Could you check a few things on this model? Use its own coordinates, in mm. A direction names the side the tool comes from. Round coordinates to 2 decimals unless told otherwise and drop trailing zeros. Write each loop counter-clockwise with the first axis right and the second up, starting at its lowest first coordinate (ties: lowest second). Pieces come first, ordered by that corner, then holes. Notation, with made-up numbers: (19, 78) -> (62, 78) arc R17 cw to (62, 84) -> close; hole circle Ø1 at (52.5, -30.75). An arc over 180 degrees is marked (long way). Answer in a Markdown table with one row per item. Add a question column.
```python
from build123d import *

# Parameters (mm, degrees)
SKETCH_W        = 40
SKETCH_H        = 35
PAD_DEPTH       = 40
SKETCH001_R     = 12.5
POCKET_DEPTH    = 40.001
SKETCH002_W     = 24.731892
SKETCH002_H     = 24.731892
POCKET001_DEPTH = 35
POCKET002_DEPTH = 35
SKETCH004_W     = 2.5
SKETCH004_H     = 30
POCKET003_DEPTH = 40.001
SKETCH005_W     = 2.5
SKETCH005_H     = 30
POCKET004_DEPTH = 21
SKETCH006_W     = 39.144078
SKETCH006_H     = 33.985684
PAD001_DEPTH    = 3
SKETCH007_W     = 18
SKETCH007_H     = 2
POCKET005_DEPTH = 5
SKETCH008_W     = 2.5
SKETCH008_H     = 15
POCKET006_DEPTH = 1.5
SKETCH009_W     = 21
SKETCH009_H     = 2.5
POCKET007_DEPTH = 1.5


with BuildPart() as part:
    # Sketch → Pad (new body)
    with BuildSketch(Plane.XY):
        with Locations((0, -2.5)):
            Rectangle(SKETCH_W, SKETCH_H)
    extrude(amount=PAD_DEPTH)

    # Sketch001 (on Face5 of Pad) → Pocket (cut, through all)
    with BuildSketch(Plane(origin=(0, 0, 0), x_dir=(1, 0, 0), z_dir=(0, 0, -1))):
        Circle(SKETCH001_R)
    extrude(amount=-POCKET_DEPTH, mode=Mode.SUBTRACT)

    # Sketch002 (on Face5 of Pocket) → Pocket001 (cut)
    with BuildSketch(Plane.XY.offset(40)):
        Rectangle(SKETCH002_W, SKETCH002_H)
    extrude(amount=-POCKET001_DEPTH, mode=Mode.SUBTRACT)

    # Sketch003 → Pocket002 (cut)
    with BuildSketch(Plane.XY.offset(40)):
        Polygon((-18.24138, 13.149356), (-15.24138, 13.149356), (-15.24138, -15.688641), (15.24138, -15.688641), (15.24138, 12.981641), (18.24138, 12.981641), (18.24138, -18.180522), (-18.24138, -18.180522), align=None)
    extrude(amount=-POCKET002_DEPTH, mode=Mode.SUBTRACT)

    # Sketch004 → Pocket003 (cut, through all)
    with BuildSketch(Plane.YZ.offset(20)):
        with Locations((-10.75, 20)):
            Rectangle(SKETCH004_W, SKETCH004_H)
        with Locations((-5.25, 20)):
            Rectangle(SKETCH004_W, SKETCH004_H)
        with Locations((0.25, 20)):
            Rectangle(SKETCH004_W, SKETCH004_H)
        with Locations((5.75, 20)):
            Rectangle(SKETCH004_W, SKETCH004_H)
    extrude(amount=-POCKET003_DEPTH, mode=Mode.SUBTRACT)

    # Sketch005 → Pocket004 (cut)
    with BuildSketch(Plane.XZ.offset(20)):
        with Locations((-5.5, 20)):
            Rectangle(SKETCH005_W, SKETCH005_H)
        with Locations((0, 20)):
            Rectangle(SKETCH005_W, SKETCH005_H)
        with Locations((5.5, 20)):
            Rectangle(SKETCH005_W, SKETCH005_H)
        with Locations((11, 20)):
            Rectangle(SKETCH005_W, SKETCH005_H)
        with Locations((-11, 20)):
            Rectangle(SKETCH005_W, SKETCH005_H)
    extrude(amount=-POCKET004_DEPTH, mode=Mode.SUBTRACT)

    # Sketch006 → Pad001 (join)
    with BuildSketch(Plane.XY.offset(40)):
        with Locations((0.008508, -2.623403)):
            Rectangle(SKETCH006_W, SKETCH006_H)
    extrude(amount=-PAD001_DEPTH)

    # Sketch007 (on Face89 of Pad001) → Pocket005 (cut)
    with BuildSketch(Plane.XY.offset(5)):
        with Locations((0, 5.022821)):
            Rectangle(SKETCH007_W, SKETCH007_H)
        Rectangle(SKETCH007_W, SKETCH007_H)
        with Locations((0, -5.022821)):
            Rectangle(SKETCH007_W, SKETCH007_H)
    extrude(amount=-POCKET005_DEPTH, mode=Mode.SUBTRACT)

    # Sketch008 (on Face117 of Pocket005) → Pocket006 (cut)
    with BuildSketch(Plane.XY.offset(40)):
        with Locations((-8.25, 0)):
            Rectangle(SKETCH008_W, SKETCH008_H)
        with Locations((8.25, 0)):
            Rectangle(SKETCH008_W, SKETCH008_H)
        with Locations((-2.75, 0)):
            Rectangle(SKETCH008_W, SKETCH008_H)
        with Locations((2.75, 0)):
            Rectangle(SKETCH008_W, SKETCH008_H)
    extrude(amount=-POCKET006_DEPTH, mode=Mode.SUBTRACT)

    # Sketch009 (on Face74 of Pocket006) → Pocket007 (cut)
    with BuildSketch(Plane(origin=(0, 0, 37), x_dir=(1, 0, 0), z_dir=(0, 0, -1))):
        with Locations((0, 4.5)):
            Rectangle(SKETCH009_W, SKETCH009_H)
        Rectangle(SKETCH009_W, SKETCH009_H)
        with Locations((0, -4.5)):
            Rectangle(SKETCH009_W, SKETCH009_H)
    extrude(amount=-POCKET007_DEPTH, mode=Mode.SUBTRACT)


solid = part.part
```
(1) I need wall thicknesses on L1, parallel to X at y = 8, z = 20; L2, parallel to Y at x = 15, z = 27; L3, parallel to Y at x = 9, z = 9.5. Which ranges of each line are inside material? Lowest first, please.
(2) Suppose I cut it at C-C, the plane z = 6.5. State how many separate pieces and enclosed holes the cut face has, then the cut area to 3 significant figures.
(3) For P1, Ø0.5, axis at x = 8.5, y = -7, coming from the +Z side; P2, Ø1, axis at x = -6, y = 4.5, coming from the -Z side, each with a flat end and sliding along its axis, tell me the tip position at first contact or that it passes through.
(4) Suppose I cut it at A-A, the plane x = 0. Please give me the cut outline in (y, z).
(5) If we mould it in two halves opening along Y, with no side actions, what happens to faces 4 (the face through (5, -5, 38.5)), 5 (the face through (19, -5, 35))? For each: pulls with the +Y half, pulls with the -Y half, needs draft (parallel to the pull), parting line crosses it, or undercut.
(6) On a 3-axis mill with a long thin cutter (end or side, diameter ignored), from which of +Z, -Z, +X, -X, +Y, -Y can I reach the whole of each face in a straight line? I mean faces 1 (the face through (8, 7.5, 39)), 2 (the face through (-14, -6.5, 20)), 3 (the face through (-10.5, 5, 38)). Say none if no direction works.
(7) Suppose I cut it at B-B, the plane y = -17. Please give me the cut outline in (x, z).
Response:
| question | item | result |
|---|---|---|
| 1 | L1 | -20 to -18.24, -15.24 to -12.37, 12.37 to 15.24, 18.24 to 20 |
| 1 | L2 | -20 to -18.18, -15.69 to -12, -9.5 to -6.5, -4 to -1, 1.5 to 4.5, 7 to 15 |
| 1 | L3 | -20 to -18.18, -15.69 to -12.37, 12.37 to 15 |
| 2 | separate pieces | 25 |
| 2 | enclosed holes | 0 |
| 2 | area | 367 mm² |
| 3 | P1 | z = 38.5 |
| 3 | P2 | z = 38.5 |
| 4 | outline | (-20, 0) -> (-12.5, 0) -> (-12.5, 5) -> (-20, 5) -> close; (-20, 35) -> (-18.18, 35) -> (-18.18, 37) -> (-15.69, 37) -> (-15.69, 35) -> (-12.5, 35) -> (-12.5, 37) -> (-5.75, 37) -> (-5.75, 38.5) -> (-3.25, 38.5) -> (-3.25, 37) -> (-1.25, 37) -> (-1.25, 38.5) -> (1.25, 38.5) -> (1.25, 37) -> (3.25, 37) -> (3.25, 38.5) -> (5.75, 38.5) -> (5.75, 37) -> (12.5, 37) -> (12.5, 0) -> (15, 0) -> (15, 40) -> (-20, 40) -> close |
| 5 | face 4 | undercut |
| 5 | face 5 | undercut |
| 6 | face 1 | +Z |
| 6 | face 2 | +X, -X |
| 6 | face 3 | -Z |
| 7 | outline | (-20, 0) -> (20, 0) -> (20, 40) -> (-20, 40) -> close; hole (-18.24, 5) -> (18.24, 5) -> (18.24, 37) -> (-18.24, 37) -> close |
